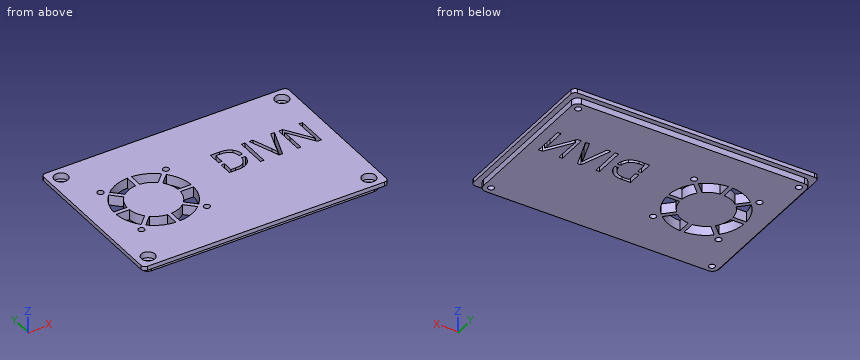
```python
from build123d import *

# Parameters (mm, degrees)
F0_W      = 120
F0_H      = 80
F0_W_2    = 115
F0_H_2    = 75
F1_DEPTH  = 2
F2_W      = 115
F2_H      = 75
F3_DEPTH  = 5
F5_R      = 3
F6_R      = 2
F7_R      = 1.5
F8_DEPTH  = 25
F9_R      = 3.35
F9_R_2    = 1.5
F10_DEPTH = 3
F11_R     = 1.5
F11_W     = 1.728515625
F11_H     = 14.873046875
F12_DEPTH = 25


with BuildPart() as f1:
    # F0 (on Top) → F1 (new body)
    with BuildSketch(Plane.XY):
        Rectangle(F0_W, F0_H)
        Rectangle(F0_W_2, F0_H_2, mode=Mode.SUBTRACT)
    extrude(amount=F1_DEPTH)


with BuildPart() as f3:
    # F2 (on face) → F3 (new body)
    with BuildSketch(Plane.XY.offset(2)):
        Rectangle(F2_W, F2_H)
    extrude(amount=-F3_DEPTH)

    # F4: union F1
    add(f1.part)

    # F5
    f5_edges = [f3.edges().sort_by_distance(p)[0] for p in [
        (-57.5, 37.5, -1.5),
        (-57.5, -37.5, -1.5),
        (57.5, -37.5, -1.5),
        (57.5, 37.5, -1.5),
    ]]
    fillet(f5_edges, radius=F5_R)

    # F6
    f6_edges = [f3.edges().sort_by_distance(p)[0] for p in [
        (60, 40, 1),
        (60, -40, 1),
        (-60, -40, 1),
        (-60, 40, 1),
    ]]
    fillet(f6_edges, radius=F6_R)

    # F7 (on face) → F8 (cut)
    with BuildSketch(Plane.XY.offset(2)):
        with Locations((-54, 34)):
            Circle(F7_R)
        with Locations((54, 34)):
            Circle(F7_R)
        with Locations((-54, -34)):
            Circle(F7_R)
        with Locations((54, -34)):
            Circle(F7_R)
    extrude(amount=-F8_DEPTH, mode=Mode.SUBTRACT)

    # F9 (on face) → F10 (cut)
    with BuildSketch(Plane.XY.offset(2)):
        with Locations((-54, 34)):
            Circle(F9_R)
        with Locations((-54, 34)):
            Circle(F9_R_2, mode=Mode.SUBTRACT)
        with Locations((54, 34)):
            Circle(F9_R)
        with Locations((54, 34)):
            Circle(F9_R_2, mode=Mode.SUBTRACT)
        with Locations((54, -34)):
            Circle(F9_R)
        with Locations((54, -34)):
            Circle(F9_R_2, mode=Mode.SUBTRACT)
        with Locations((-54, -34)):
            Circle(F9_R)
        with Locations((-54, -34)):
            Circle(F9_R_2, mode=Mode.SUBTRACT)
    extrude(amount=-F10_DEPTH, mode=Mode.SUBTRACT)

    # F11 (on face) → F12 (cut)
    with BuildSketch(Plane.XY.offset(2)):
        with BuildLine():
            Line((-17.5400642056, 1), (-11.026334039, 1))
            ThreePointArc((-11.026334039, 1), (-12.4462888823, 7.2709852149), (-15.8764853538, 12.7093010838))
            Line((-15.8764853538, 12.7093010838), (-20.4823881255, 8.1033983122))
            ThreePointArc((-20.4823881255, 8.1033983122), (-18.4515058436, 4.7835429046), (-17.5400642056, 1))
        make_face()
        with Locations((-14, 16)):
            Circle(F11_R)
        with BuildLine():
            Line((-21.8966016878, 9.5176118745), (-17.2906989162, 14.1235146462))
            ThreePointArc((-17.2906989162, 14.1235146462), (-22.7290147851, 17.5537111177), (-29, 18.973665961))
            Line((-29, 18.973665961), (-29, 12.4599357944))
            ThreePointArc((-29, 12.4599357944), (-25.2164570954, 11.5484941564), (-21.8966016878, 9.5176118745))
        make_face()
        with BuildLine():
            Line((-31, 12.4599357944), (-31, 18.973665961))
            ThreePointArc((-31, 18.973665961), (-37.2709852149, 17.5537111177), (-42.7093010838, 14.1235146462))
            Line((-42.7093010838, 14.1235146462), (-38.1033983122, 9.5176118745))
            ThreePointArc((-38.1033983122, 9.5176118745), (-34.7835429046, 11.5484941564), (-31, 12.4599357944))
        make_face()
        with BuildLine():
            Line((-39.5176118745, 8.1033983122), (-44.1235146462, 12.7093010838))
            ThreePointArc((-44.1235146462, 12.7093010838), (-47.5537111177, 7.2709852149), (-48.973665961, 1))
            Line((-48.973665961, 1), (-42.4599357944, 1))
            ThreePointArc((-42.4599357944, 1), (-41.5484941564, 4.7835429046), (-39.5176118745, 8.1033983122))
        make_face()
        with BuildLine():
            ThreePointArc((-48.973665961, -1), (-47.5537111177, -7.2709852149), (-44.1235146462, -12.7093010838))
            Line((-44.1235146462, -12.7093010838), (-39.5176118745, -8.1033983122))
            ThreePointArc((-39.5176118745, -8.1033983122), (-41.5484941564, -4.7835429046), (-42.4599357944, -1))
            Line((-42.4599357944, -1), (-48.973665961, -1))
        make_face()
        with BuildLine():
            ThreePointArc((-42.7093010838, -14.1235146462), (-37.2709852149, -17.5537111177), (-31, -18.973665961))
            Line((-31, -18.973665961), (-31, -12.4599357944))
            ThreePointArc((-31, -12.4599357944), (-34.7835429046, -11.5484941564), (-38.1033983122, -9.5176118745))
            Line((-38.1033983122, -9.5176118745), (-42.7093010838, -14.1235146462))
        make_face()
        with BuildLine():
            ThreePointArc((-29, -18.973665961), (-22.7290147851, -17.5537111177), (-17.2906989162, -14.1235146462))
            Line((-17.2906989162, -14.1235146462), (-21.8966016878, -9.5176118745))
            ThreePointArc((-21.8966016878, -9.5176118745), (-25.2164570954, -11.5484941564), (-29, -12.4599357944))
            Line((-29, -12.4599357944), (-29, -18.973665961))
        make_face()
        with BuildLine():
            ThreePointArc((-15.8764853538, -12.7093010838), (-12.4462888823, -7.2709852149), (-11.026334039, -1))
            Line((-11.026334039, -1), (-17.5400642056, -1))
            ThreePointArc((-17.5400642056, -1), (-18.4515058436, -4.7835429046), (-20.4823881255, -8.1033983122))
            Line((-20.4823881255, -8.1033983122), (-15.8764853538, -12.7093010838))
        make_face()
        with Locations((-14, -16)):
            Circle(F11_R)
        with Locations((-46, -16)):
            Circle(F11_R)
        with Locations((-46, 16)):
            Circle(F11_R)
        with Locations((23.0973307292, 7.4365234375)):
            Rectangle(F11_W, F11_H)
        with BuildLine():
            Line((38.3951822917, 14.873046875), (36.5364583333, 14.873046875))
            Line((36.5364583333, 14.873046875), (33.1380208333, 5.3092447917))
            add(Edge.make_bspline(
                [(32.1809895833, 2.0247395833), (32.548828125, 3.671875), (33.1380208333, 5.3092447917)],
                knots=[0, 0, 0, 1, 1, 1], degree=2))
            add(Edge.make_bspline(
                [(31.2467447917, 5.2506510417), (31.8359375, 3.5904947917), (32.1809895833, 2.0247395833)],
                knots=[0, 0, 0, 1, 1, 1], degree=2))
            Line((31.2467447917, 5.2506510417), (27.8287760417, 14.873046875))
            Line((27.8287760417, 14.873046875), (25.99609375, 14.873046875))
            Line((25.99609375, 14.873046875), (31.328125, 0))
            Line((31.328125, 0), (33.037109375, 0))
            Line((33.037109375, 0), (38.3951822917, 14.873046875))
        make_face()
        with BuildLine():
            Line((50.0846354167, 0), (52.0572916667, 0))
            Line((52.0572916667, 0), (52.0572916667, 14.873046875))
            Line((52.0572916667, 14.873046875), (50.439453125, 14.873046875))
            Line((50.439453125, 14.873046875), (50.439453125, 6.337890625))
            add(Edge.make_bspline(
                [(50.4915364583, 4.2057291667), (50.419921875, 5.6966145833), (50.439453125, 6.337890625)],
                knots=[0, 0, 0, 1, 1, 1], degree=2))
            add(Edge.make_bspline(
                [(50.5826822917, 2.44140625), (50.5631510417, 2.71484375), (50.4915364583, 4.2057291667)],
                knots=[0, 0, 0, 1, 1, 1], degree=2))
            Line((50.5826822917, 2.44140625), (50.5013020833, 2.44140625))
            Line((50.5013020833, 2.44140625), (42.392578125, 14.873046875))
            Line((42.392578125, 14.873046875), (40.439453125, 14.873046875))
            Line((40.439453125, 14.873046875), (40.439453125, 0))
            Line((40.439453125, 0), (42.0377604167, 0))
            Line((42.0377604167, 0), (42.0377604167, 8.4537760417))
            add(Edge.make_bspline(
                [(41.875, 12.48046875), (42.0377604167, 10.283203125), (42.0377604167, 8.4537760417)],
                knots=[0, 0, 0, 1, 1, 1], degree=2))
            Line((41.875, 12.48046875), (41.9563802083, 12.48046875))
            Line((41.9563802083, 12.48046875), (50.0846354167, 0))
        make_face()
        with BuildLine():
            Line((7.0442708333, 14.873046875), (7.0442708333, 8.5))
            Line((7.0442708333, 8.5), (8.7727864583, 8.5))
            Line((8.7727864583, 8.5), (8.7727864583, 13.3756510417))
            Line((8.7727864583, 13.3756510417), (11.2858072917, 13.3756510417))
            add(Edge.make_bspline(
                [(15.6266276042, 11.9010416667), (14.1666666667, 13.3756510417), (11.2858072917, 13.3756510417)],
                knots=[0, 0, 0, 1, 1, 1], degree=2))
            add(Edge.make_bspline(
                [(17.0409949545, 8.5), (16.8285868821, 10.6870225966), (15.6266276042, 11.9010416667)],
                knots=[0.1767181936, 0.1767181936, 0.1767181936, 1, 1, 1], degree=2))
            Line((17.0409949545, 8.5), (18.8795207861, 8.5))
            add(Edge.make_bspline(
                [(16.9938151042, 12.9508463542), (18.6511564201, 11.2935050382), (18.8795207861, 8.5)],
                knots=[0, 0, 0, 0.8622104187, 0.8622104187, 0.8622104187], degree=2))
            add(Edge.make_bspline(
                [(11.6015625, 14.873046875), (15.0716145833, 14.873046875), (16.9938151042, 12.9508463542)],
                knots=[0, 0, 0, 1, 1, 1], degree=2))
            Line((11.6015625, 14.873046875), (7.0442708333, 14.873046875))
        make_face()
        with BuildLine():
            Line((8.7727864583, 6.5), (7.0442708333, 6.5))
            Line((7.0442708333, 6.5), (7.0442708333, 0))
            Line((7.0442708333, 0), (11.1653645833, 0))
            add(Edge.make_bspline(
                [(16.9173177083, 1.9482421875), (14.9186197917, 0), (11.1653645833, 0)],
                knots=[0, 0, 0, 1, 1, 1], degree=2))
            add(Edge.make_bspline(
                [(18.8699305641, 6.5), (18.6125191418, 3.600649448), (16.9173177083, 1.9482421875)],
                knots=[0.1518471004, 0.1518471004, 0.1518471004, 1, 1, 1], degree=2))
            Line((18.8699305641, 6.5), (17.0370247976, 6.5))
            add(Edge.make_bspline(
                [(15.5289713542, 3.0159505208), (16.8087372513, 4.2662965123), (17.0370247976, 6.5)],
                knots=[0, 0, 0, 0.8216177296, 0.8216177296, 0.8216177296], degree=2))
            add(Edge.make_bspline(
                [(10.87890625, 1.494140625), (13.9713541667, 1.494140625), (15.5289713542, 3.0159505208)],
                knots=[0, 0, 0, 1, 1, 1], degree=2))
            Line((10.87890625, 1.494140625), (8.7727864583, 1.494140625))
            Line((8.7727864583, 1.494140625), (8.7727864583, 6.5))
        make_face()
    extrude(amount=-F12_DEPTH, mode=Mode.SUBTRACT)


solid = f3.part
```
Here's how the part is built. I have some questions about the finished solid (model axes, mm). Round coordinates to 2 decimals unless told otherwise and drop trailing zeros. Order: outer loops, then holes, each group sorted by start corner. A loop starts at its lowest first (then second) coordinate and runs counter-clockwise, first axis right, second up. Notation, with made-up numbers: (10, 25) -> (68, 25) arc R31 cw to (68, 63) -> close; hole circle Ø10 at (26.25, 75). An arc over 180 degrees is marked (long way). Use a Markdown table: item, result. Add a question column.
(1) Suppose I cut it at D-D, the plane z = 0.9. Count the separate pieces of the cut face and the enclosed holes in it, and give its area (3 significant figures).
(2) Suppose I cut it at B-B, the plane y = -24. Please give me the cut outline in (x, z).
(3) Suppose I cut it at A-A, the plane x = -46. Please give me the cut outline in (y, z).
(4) Suppose I cut it at C-C, the plane x = 46.5. Please give me the cut outline in (y, z).
(5) I need wall thicknesses on line 1 along X through (y, z) = (-13.5, -0.9); line 2 along X through (y, z) = (-15, 1); line 3 along Y through (x, z) = (-46, -1.75). Which ranges of each line are inside material? Lowest first, please.
(6) For pin 1 Ø2 at (x, z) = (51, -0.5) entering from +Y; pin 2 Ø3.5 at (x, y) = (-54.5, 34) entering from +Z; pin 3 Ø1 at (y, z) = (-6.5, -1) entering from -X; pin 4 Ø1.5 at (y, z) = (9, -1.5) entering from +X, each with a flat end and sliding along its axis, tell me the tip position at first contact or that it passes through.
Verdict:
| question | item | result |
|---|---|---|
| 1 | separate pieces | 1 |
| 1 | enclosed holes | 21 |
| 1 | area | 8,680 mm2 |
| 2 | outline | (-60, 0) -> (-57.5, 0) -> (-57.5, -3) -> (57.5, -3) -> (57.5, 0) -> (60, 0) -> (60, 2) -> (-60, 2) -> close |
| 3 | outline | (-40, 0) -> (-37.5, 0) -> (-37.5, -3) -> (-17.5, -3) -> (-17.5, 2) -> (-40, 2) -> close; (-14.5, -3) -> (-10.25, -3) -> (-10.25, 2) -> (-14.5, 2) -> close; (-1, -3) -> (1, -3) -> (1, 2) -> (-1, 2) -> close; (10.25, -3) -> (14.5, -3) -> (14.5, 2) -> (10.25, 2) -> close; (17.5, -3) -> (37.5, -3) -> (37.5, 0) -> (40, 0) -> (40, 2) -> (17.5, 2) -> close |
| 4 | outline | (-40, 0) -> (-37.5, 0) -> (-37.5, -3) -> (5.5, -3) -> (5.5, 2) -> (-40, 2) -> close; (8.58, -3) -> (37.5, -3) -> (37.5, 0) -> (40, 0) -> (40, 2) -> (8.58, 2) -> close |
| 5 | line 1 | -57.5 to -42.09, -31 to -29, -17.91 to 57.5 |
| 5 | line 2 | -60 to -47.12, -44.88 to -41.66, -31 to -29, -18.34 to -15.12, -12.88 to 60 |
| 5 | line 3 | -37.5 to -17.5, -14.5 to -10.25, -1 to 1, 10.25 to 14.5, 17.5 to 37.5 |
| 6 | pin 1 | y = 40 |
| 6 | pin 2 | z = -1 |
| 6 | pin 3 | x = -57.5 |
| 6 | pin 4 | x = 57.5 |
